from build123d import *

# Parameters (mm, degrees)
SKETCH1_R           = 4.191
SKETCH1_R_2         = 3.3655
SKETCH1_R_3         = 7.8105
BOSS_EXTRUDE1_DEPTH = 3.175
CUT_EXTRUDE1_DEPTH  = 6.35
FILLET5_R           = 7.62
FILLET6_R           = 3.175


with BuildPart() as part:
    # Sketch1 → Boss-Extrude1 (new body)
    # profile 1 of 2: a face of its own
    with BuildSketch(Plane.XY):
        with BuildLine():
            ThreePointArc((-10.16, 168.656), (-1.971422335, 178.622899918), (9.394939759, 172.523907306))
            Line((9.394939759, 172.523907306), (55.423036695, 60.724124173))
            ThreePointArc((55.423036695, 60.724124173), (56.188096936, 56.856216867), (55.423036695, 52.988309562))
            Line((55.423036695, 52.988309562), (8.177790267, -11.326281223))
            ThreePointArc((8.177790267, -11.326281223), (-6.360706327, -12.437938536), (-13.97, 0))
            ThreePointArc((-13.97, 0), (19.399795867, 83.617198889), (-10.16, 168.656))
        make_face()
        with Locations((0, 168.656)):
            Circle(SKETCH1_R, mode=Mode.SUBTRACT)
        with Locations((46.028096936, 56.856216867)):
            Circle(SKETCH1_R_2, mode=Mode.SUBTRACT)
        Circle(SKETCH1_R_3, mode=Mode.SUBTRACT)
    # profile 2 of 2: a face of its own
    with BuildSketch(Plane.XY):
        with BuildLine():
            ThreePointArc((-5.736787087, 10.049695637), (-8.361074259, 6.616758401), (-11.099067746, 3.27380568))
            ThreePointArc((-11.099067746, 3.27380568), (-1.65388195, -11.453025058), (11.571823904, 0))
            ThreePointArc((11.571823904, 0), (5.810422469, 10.007302294), (-5.736787087, 10.049695637))
        make_face()
        Circle(SKETCH1_R_3, mode=Mode.SUBTRACT)
    extrude(amount=BOSS_EXTRUDE1_DEPTH)

    # Sketch2 → Cut-Extrude1 (cut)
    with BuildSketch(Plane.XY.offset(3.175)):
        with BuildLine():
            ThreePointArc((24.342369565, 93.274569778), (24.372628405, 80.404838249), (23.166725616, 67.591692511))
            Line((23.166725616, 67.591692511), (43.590488936, 62.925500803))
            ThreePointArc((43.590488936, 62.925500803), (46.410316451, 63.385539075), (49.157207608, 62.599631066))
            Line((49.157207608, 62.599631066), (34.133316244, 99.091858815))
            Line((34.133316244, 99.091858815), (24.342369565, 93.274569778))
        make_face()
        with BuildLine():
            Line((39.723792881, 58.598023584), (22.350976776, 62.56716919))
            ThreePointArc((22.350976776, 62.56716919), (18.436727595, 46.655838158), (12.607589722, 31.342022385))
            Line((12.607589722, 31.342022385), (47.239535948, 50.428888047))
            ThreePointArc((47.239535948, 50.428888047), (41.214780777, 52.427884471), (39.723792881, 58.598023584))
        make_face()
        with BuildLine():
            Line((40.079895195, 40.682524127), (8.679618073, 23.376743294))
            ThreePointArc((8.679618073, 23.376743294), (5.069193292, 17.049607217), (1.119884547, 10.928269252))
            ThreePointArc((1.119884547, 10.928269252), (7.805850235, 7.729806748), (10.938708503, 1.012850693))
            Line((10.938708503, 1.012850693), (40.079895195, 40.682524127))
        make_face()
    extrude(amount=-CUT_EXTRUDE1_DEPTH, mode=Mode.SUBTRACT)

    # Fillet5
    fillet5_edges = [part.edges().sort_by_distance(p)[0] for p in [
        (55.423036695, 52.988309562, 1.5875),
        (8.177790267, -11.326281223, 1.5875),
        (-13.97, 0, 1.5875),
        (-10.16, 168.656, 1.5875),
    ]]
    fillet(fillet5_edges, radius=FILLET5_R)

    # Fillet6
    fillet6_edges = [part.edges().sort_by_distance(p)[0] for p in [
        (24.342369565, 93.274569778, 1.5875),
        (34.133316244, 99.091858815, 1.5875),
        (49.157207608, 62.599631066, 1.5875),
        (43.590488936, 62.925500803, 1.5875),
        (23.166725616, 67.591692511, 1.5875),
        (8.679618073, 23.376743294, 1.5875),
        (40.079895195, 40.682524127, 1.5875),
        (10.938708503, 1.012850693, 1.5875),
        (1.119884547, 10.928269252, 1.5875),
        (22.350976776, 62.56716919, 1.5875),
        (39.723792881, 58.598023584, 1.5875),
        (47.239535948, 50.428888047, 1.5875),
        (12.607589722, 31.342022385, 1.5875),
    ]]
    fillet(fillet6_edges, radius=FILLET6_R)


solid = part.part
Source: CAD feature listing. Evaluate the final solid. Frame: model axes, mm. A direction names the side the tool comes from. Coordinates: 2 decimals unless noted, no trailing zeros. Order: outer loops, then holes, each group sorted by start corner. A loop starts at its lowest first (then second) coordinate and runs counter-clockwise, first axis right, second up.
Item 1: Set-up query: faces 4 (the face through (19.296, 49.52, 1.61)), 5 (the face through (55.583, 53.58, 1.61)). Return all of +Z, -Z, +X, -X, +Y, -Y with unobstructed straight access to the full face (end or side cutting, diameter ignored); none if empty.
Output values:
face 4: +Z, -Z
face 5: +Z, -Z, +X, -Y
Item 2: Material intervals for line 1 (Y direction, x = 0, z = 2.5) (1 decimal); line 2 (Y direction, x = 8, z = 2.95); line 3 (Y direction, x = 27.5, z = 0.3), sorted ascending.
Output values:
line 1: y = -14 to -7.8, 7.8 to 18.5, 154.5 to 164.5, 172.8 to 178.8
line 2: y = -11.31 to 7.53, 22.12 to 33.48, 139.57 to 174.92
line 3: y = 14.98 to 23.56, 33.75 to 39.55, 61.39 to 66.6, 95.15 to 128.55
Item 3: Pull-direction query (X, two-part tool) for faces 1 (the face through (24.114, 68.19, 1.565)), 2 (the face through (32.176, 21.342, 1.565)), 3 (the face through (1.806, 178.654, 1.565)); classes: pulls with the +X half, pulls with the -X half, needs draft (parallel to the pull), parting line crosses it, or undercut.
Output values:
face 1: undercut
face 2: pulls with the +X half
face 3: parting line crosses it
Item 4: Cut plane C-C (y = 154). Return loops of the section in (x, z) (3 decimals), plus the area to 3 significant figures.
Output values:
outline: (0.339, 0) - (17.021, 0) - (17.021, 3.175) - (0.339, 3.175) - close
area: 53.0 mm2
Item 5: Cut plane B-B (z = 2.3). Count the separate pieces of the cut face and the enclosed holes in it, plus the area to 3 significant figures.
Output values:
separate pieces: 1
enclosed holes: 6
area: 3,130 mm2
Item 6: First-contact query: P1, Ø1.5, axis at y = 77.5, z = 1, coming from the -X side; P2, Ø14, axis at x = 0, y = 0, coming from the -Z side; P3, Ø1.5, axis at x = 23.5, z = 1.5, coming from the +Y side. Flat tips, straight axial feed; report the tip coordinate or a pass-through.
Output values:
P1: stops at x = 19.06
P2: passes through
P3: stops at y = 140.09
Item 7: Cut plane A-A (x = 0). Return loops of the section in (y, z) (1 decimal).
Output values:
outline: (-14, 0) - (-7.8, 0) - (-7.8, 3.2) - (-14, 3.2) - close; (7.8, 0) - (18.5, 0) - (18.5, 3.2) - (7.8, 3.2) - close; (154.5, 0) - (164.5, 0) - (164.5, 3.2) - (154.5, 3.2) - close; (172.8, 0) - (178.8, 0) - (178.8, 3.2) - (172.8, 3.2) - close
